Part print with two shaded views. Sizes in mm from the minimum x, y, z corner. A direction names the side the tool comes from. Give positions to 0.01 mm unless a question says otherwise; leave off trailing zeros. Loops run counter-clockwise (first coordinate to the right, second up) from the corner with the lowest first, then second, coordinate; pieces in that order, holes last. Notation, with made-up numbers: M 23.5,19.5 L 47.5,19.5 A29 ccw 47.5,47.5 Z; hole C 86,7.25 d5. An arc over 180 degrees is marked long. Answer as a JSON object with one key per item and string values. Group by question number.
1. 3-axis set-ups, long thin cutter, end or side, ignore diameter. For the marked faces 1, 2 and 3: which of +Z, -Z, +X, -X, +Y, -Y reach the whole face in a straight line?
2. Slice it at C-C (x = 69). List the corners of the cut face in (y, z) (3 decimals).
3. Drop flat-ended pins along their axis: pin 1 Ø2 at (x, z) = (15.5, 3.5) entering from +Y; pin 2 Ø4 at (x, z) = (34.5, 7) entering from -Y (3 decimals); pin 3 Ø6 at (x, z) = (45, 10.5) entering from +Y. Give the stop position or say it passes through.
4. Drill centre lines: line 1 along X through (y, z) = (9.75, 5.5); line 2 along X through (y, z) = (8.75, 12.5); line 3 along Z through (x, y) = (20, 9.25). Where is each one in solid material? Low to high. Write a range as [from, to].
5. Slice it at A-A (z = 6.48). List the corners of the cut face in (x, y) (3 decimals).
6. Slice it at D-D (x = 41). List the corners of the cut face in (y, z) (3 decimals).
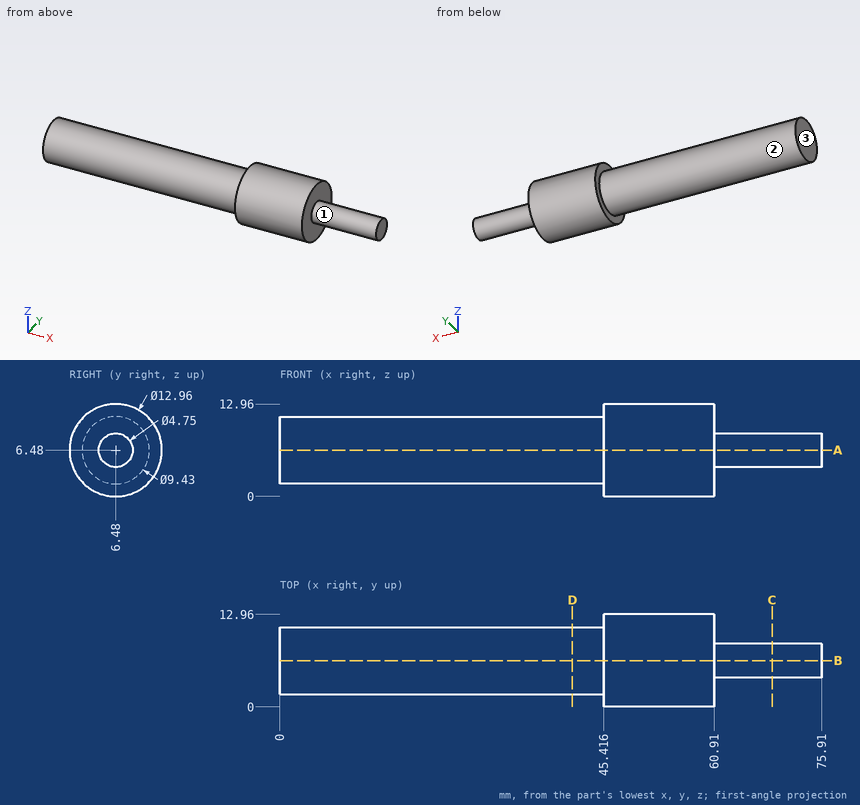
Established:
{
 "1": {"face 1": "+X", "face 2": "-X", "face 3": "+Z, -Z, -X, +Y, -Y"},
 "2": {"outline": "C 6.48,6.48 d4.75"},
 "3": {"pin 1": "stops at y = 10.76", "pin 2": "stops at y = 1.765", "pin 3": "stops at y = 12.87"},
 "4": {"line 1": "x = [0, 60.91]", "line 2": "x = [45.42, 60.91]", "line 3": "z = [2.66, 10.3]"},
 "5": {"outline": "M 0,1.765 L 45.416,1.765 L 45.416,0 L 60.91,0 L 60.91,4.105 L 75.91,4.105 L 75.91,8.855 L 60.91,8.855 L 60.91,12.96 L 45.416,12.96 L 45.416,11.195 L 0,11.195 Z"},
 "6": {"outline": "C 6.48,6.48 d9.43"}
}
